Autodesk Inventor part; units mm, degrees
ref_plane "YZ Plane" through (0, 0, 0) normal (1, 0, 0) x (0, 1, 0)
ref_plane "XZ Plane" through (0, 0, 0) normal (0, 1, 0) x (-1, 0, 0)
ref_plane "XY Plane" through (0, 0, 0) normal (0, 0, 1) x (1, 0, 0)
sketch "Sketch1" plane through (0, 0, 0) normal (0, 1, 0) x (-1, 0, 0)
  arc A0 (4.5962, 6.7175) -> (6.7175, 4.5962) centre (5.6569, 5.6569) ccw
  line L0 (5.6569, 7.7782) -> (4.5962, 6.7175)
  arc A1 (7.7782, 5.6569) -> (5.6569, 7.7782) centre (6.7175, 6.7175) ccw
  line L1 (6.7175, 4.5962) -> (7.7782, 5.6569)
  circle A2 centre (0, 0) radius 3
  circle A3 centre (0, -124.0736) radius 1.5
  circle A4 centre (0, -145.2868) radius 4
  arc A5 (-4.5962, -6.7175) -> (-6.7175, -4.5962) centre (-5.6569, -5.6569) ccw
  line L2 (-5.6569, -7.7782) -> (-4.5962, -6.7175)
  arc A6 (-7.7782, -5.6569) -> (-5.6569, -7.7782) centre (-6.7175, -6.7175) ccw
  line L3 (-6.7175, -4.5962) -> (-7.7782, -5.6569)
  line L4 (-20, 5.4953) -> (-20, -6.6667)
  arc A7 (-20, -6.6667) -> (-18, -12.6667) centre (-10, -6.6667) ccw
  line L5 (-18, -12.6667) -> (-14.5, -17.3333)
  arc A8 (-12.5, -23.3333) -> (-14.5, -17.3333) centre (-22.5, -23.3333) ccw
  line L6 (-12.5, -23.3333) -> (-12.5, -134.321)
  arc A9 (-12.5, -134.321) -> (-12.2297, -138.6622) centre (22.5, -134.321) ccw
  line L7 (-12.2297, -138.6622) -> (-10, -156.5)
  line L8 (-10, -156.5) -> (-10, -166.5)
  line L9 (-10, -166.5) -> (0, -166.5)
  line L10 (0, -166.5) -> (0, -156.5)
  line L11 (0, -156.5) -> (10, -156.5)
  line L12 (10, -156.5) -> (12.2297, -138.6622)
  arc A10 (12.2297, -138.6622) -> (12.5, -134.321) centre (-22.5, -134.321) ccw
  line L13 (12.5, -134.321) -> (12.5, -23.3333)
  arc A11 (14.5, -17.3333) -> (12.5, -23.3333) centre (22.5, -23.3333) ccw
  line L14 (14.5, -17.3333) -> (18, -12.6667)
  arc A12 (18, -12.6667) -> (20, -6.6667) centre (10, -6.6667) ccw
  line L15 (20, -6.6667) -> (20, 5.4953)
  arc A13 (20, 5.4953) -> (16.6262, 12.9849) centre (10, 5.4953) ccw
  line L16 (16.6262, 12.9849) -> (6.6262, 21.8321)
  arc A14 (6.6262, 21.8321) -> (-6.6262, 21.8321) centre (0, 14.3426) ccw
  line L17 (-6.6262, 21.8321) -> (-16.6262, 12.9849)
  arc A15 (-16.6262, 12.9849) -> (-20, 5.4953) centre (-10, 5.4953) ccw
  arc A16 (-6.7175, 4.5962) -> (-4.5962, 6.7175) centre (-5.6569, 5.6569) ccw
  line L18 (-7.7782, 5.6569) -> (-6.7175, 4.5962)
  arc A17 (-5.6569, 7.7782) -> (-7.7782, 5.6569) centre (-6.7175, 6.7175) ccw
  line L19 (-4.5962, 6.7175) -> (-5.6569, 7.7782)
  arc A18 (6.7175, -4.5962) -> (4.5962, -6.7175) centre (5.6569, -5.6569) ccw
  line L20 (7.7782, -5.6569) -> (6.7175, -4.5962)
  arc A19 (5.6569, -7.7782) -> (7.7782, -5.6569) centre (6.7175, -6.7175) ccw
  line L21 (4.5962, -6.7175) -> (5.6569, -7.7782)
  circle A20 centre (6, -136.5) radius 1.5
  circle A21 centre (-6, -136.5) radius 1.5
  point P0 (18, -12.6667)
  point P1 (16.6262, 12.9849)
  point P2 (6.6262, 21.8321)
  point P3 (-6.6262, 21.8321)
  point P4 (-16.6262, 12.9849)
  point P5 (-18, -12.6667)
  point P6 (-14.5, -17.3333)
  point P7 (-12.5, -23.3333)
  point P8 (-12.5, -134.321)
  point P9 (-12.2297, -138.6622)
  point P10 (12.2297, -138.6622)
  point P11 (12.5, -134.321)
  point P12 (12.5, -23.3333)
  point P13 (14.5, -17.3333)
  point P14 (-6.7175, -4.5962)
  point P15 (-4.5962, -6.7175)
  point P16 (-5.6569, -7.7782)
  point P17 (-7.7782, -5.6569)
  point P18 (7.7782, 5.6569)
  point P19 (6.7175, 4.5962)
  point P20 (4.5962, 6.7175)
  point P21 (5.6569, 7.7782)
  point P22 (-5.6569, 7.7782)
  point P23 (-4.5962, 6.7175)
  point P24 (-6.7175, 4.5962)
  point P25 (-7.7782, 5.6569)
  point P26 (6.7175, -4.5962)
  point P27 (7.7782, -5.6569)
  point P28 (5.6569, -7.7782)
  point P29 (4.5962, -6.7175)
extrude "Extrusion1" add sketch "Sketch1" along normal blind 6
sketch "Sketch2" plane through (0, 6, 0) normal (0, 1, 0) x (1, 0, 0)
  line L0 (20, -5.4953) -> (20, 6.6667)
  arc A0 (20, 6.6667) -> (18, 12.6667) centre (10, 6.6667) ccw
  line L1 (18, 12.6667) -> (14.5, 17.3333)
  arc A1 (12.5, 23.3333) -> (14.5, 17.3333) centre (22.5, 23.3333) ccw
  line L2 (12.5, 23.3333) -> (12.5, 134.321)
  arc A2 (12.5, 134.321) -> (12.2297, 138.6622) centre (-22.5, 134.321) ccw
  line L3 (12.2297, 138.6622) -> (10, 156.5)
  line L4 (10, 156.5) -> (10, 166.5)
  line L5 (10, 166.5) -> (0, 166.5)
  line L6 (0, 166.5) -> (0, 156.5)
  line L7 (0, 156.5) -> (-10, 156.5)
  line L8 (-10, 156.5) -> (-12.2297, 138.6622)
  arc A3 (-12.2297, 138.6622) -> (-12.5, 134.321) centre (22.5, 134.321) ccw
  line L9 (-12.5, 134.321) -> (-12.5, 23.3333)
  arc A4 (-14.5, 17.3333) -> (-12.5, 23.3333) centre (-22.5, 23.3333) ccw
  line L10 (-14.5, 17.3333) -> (-18, 12.6667)
  arc A5 (-18, 12.6667) -> (-20, 6.6667) centre (-10, 6.6667) ccw
  line L11 (-20, 6.6667) -> (-20, -5.4953)
  arc A6 (-20, -5.4953) -> (-16.6262, -12.9849) centre (-10, -5.4953) ccw
  line L12 (-16.6262, -12.9849) -> (-6.6262, -21.8321)
  arc A7 (-6.6262, -21.8321) -> (6.6262, -21.8321) centre (0, -14.3426) ccw
  line L13 (6.6262, -21.8321) -> (16.6262, -12.9849)
  arc A8 (16.6262, -12.9849) -> (20, -5.4953) centre (10, -5.4953) ccw
  circle A9 centre (0, 0) radius 3
  circle A10 centre (0, 145.2868) radius 4
  circle A11 centre (-6, 136.5) radius 1.5
  circle A12 centre (6, 136.5) radius 1.5
  circle A13 centre (0, 124.0736) radius 1.5
  line L14 (7.7782, 5.6569) -> (6.7175, 4.5962)
  arc A14 (4.5962, 6.7175) -> (6.7175, 4.5962) centre (5.6569, 5.6569) ccw
  line L15 (4.5962, 6.7175) -> (5.6569, 7.7782)
  arc A15 (7.7782, 5.6569) -> (5.6569, 7.7782) centre (6.7175, 6.7175) ccw
  line L16 (-7.7782, -5.6569) -> (-6.7175, -4.5962)
  arc A16 (-4.5962, -6.7175) -> (-6.7175, -4.5962) centre (-5.6569, -5.6569) ccw
  line L17 (-4.5962, -6.7175) -> (-5.6569, -7.7782)
  arc A17 (-7.7782, -5.6569) -> (-5.6569, -7.7782) centre (-6.7175, -6.7175) ccw
  arc A18 (5.6569, -7.7782) -> (7.7782, -5.6569) centre (6.7175, -6.7175) ccw
  line L18 (5.6569, -7.7782) -> (4.5962, -6.7175)
  arc A19 (6.7175, -4.5962) -> (4.5962, -6.7175) centre (5.6569, -5.6569) ccw
  line L19 (6.7175, -4.5962) -> (7.7782, -5.6569)
  line L20 (-6.7175, 4.5962) -> (-7.7782, 5.6569)
  arc A20 (-5.6569, 7.7782) -> (-7.7782, 5.6569) centre (-6.7175, 6.7175) ccw
  line L21 (-5.6569, 7.7782) -> (-4.5962, 6.7175)
  arc A21 (-6.7175, 4.5962) -> (-4.5962, 6.7175) centre (-5.6569, 5.6569) ccw
  line L22 (18.6141, -15.2318) -> (8.6141, -24.079)
  arc A22 (-8.6141, -24.079) -> (8.6141, -24.079) centre (0, -14.3426) ccw
  line L23 (-8.6141, -24.079) -> (-18.6141, -15.2318)
  arc A23 (-23, -5.4953) -> (-18.6141, -15.2318) centre (-10, -5.4953) ccw
  line L24 (-23, -5.4953) -> (-23, 6.6667)
  arc A24 (-20.4, 14.4667) -> (-23, 6.6667) centre (-10, 6.6667) ccw
  line L25 (-20.4, 14.4667) -> (-12.5, 25)
  line L26 (-15.5, 23.3333) -> (-15.5, 134.321)
  arc A25 (-15.2066, 139.0343) -> (-15.5, 134.321) centre (22.5, 134.321) ccw
  line L27 (-15.2066, 139.0343) -> (-12.6483, 159.5)
  line L28 (-12.6483, 159.5) -> (-3, 159.5)
  line L29 (-3, 159.5) -> (-3, 169.5)
  line L30 (-3, 169.5) -> (13, 169.5)
  line L31 (13, 169.5) -> (13, 156.6868)
  line L32 (13, 156.6868) -> (15.2066, 139.0343)
  arc A26 (15.5, 134.321) -> (15.2066, 139.0343) centre (-22.5, 134.321) ccw
  line L33 (15.5, 134.321) -> (15.5, 23.3333)
  line L34 (12.5, 25) -> (20.4, 14.4667)
  arc A27 (23, 6.6667) -> (20.4, 14.4667) centre (10, 6.6667) ccw
  line L35 (23, 6.6667) -> (23, -5.4953)
  arc A28 (18.6141, -15.2318) -> (23, -5.4953) centre (10, -5.4953) ccw
  dimension "d2" = 3
extrude "Extrusion2" add sketch "Sketch2" against normal blind 6 contours L0 A0 L1 A1 L2 L34 A27 L35 A28 L22 A22 L23 A23 L24 A24 L25 L9 A4 L10 A5 L11 A6 L12 A7 L13 A8
sketch "Sketch3" plane through (0, 6, 0) normal (0, 1, 0) x (1, 0, 0)
  line L0 (12.5, 25) -> (12.5, 134.321)
  arc A0 (12.5, 134.321) -> (12.2297, 138.6622) centre (-22.5, 134.321) ccw
  line L1 (12.2297, 138.6622) -> (10, 156.5)
  line L2 (10, 156.5) -> (10, 166.5)
  line L3 (10, 166.5) -> (0, 166.5)
  line L4 (0, 166.5) -> (0, 156.5)
  line L5 (0, 156.5) -> (-10, 156.5)
  line L6 (-10, 156.5) -> (-12.2297, 138.6622)
  arc A1 (-12.2297, 138.6622) -> (-12.5, 134.321) centre (22.5, 134.321) ccw
  line L7 (-12.5, 134.321) -> (-12.5, 25)
  circle A2 centre (0, 0) radius 3
  circle A3 centre (0, 145.2868) radius 4
  circle A4 centre (-6, 136.5) radius 1.5
  circle A5 centre (6, 136.5) radius 1.5
  circle A6 centre (0, 124.0736) radius 1.5
  line L8 (7.7782, 5.6569) -> (6.7175, 4.5962)
  arc A7 (4.5962, 6.7175) -> (6.7175, 4.5962) centre (5.6569, 5.6569) ccw
  line L9 (4.5962, 6.7175) -> (5.6569, 7.7782)
  arc A8 (7.7782, 5.6569) -> (5.6569, 7.7782) centre (6.7175, 6.7175) ccw
  line L10 (-7.7782, -5.6569) -> (-6.7175, -4.5962)
  arc A9 (-4.5962, -6.7175) -> (-6.7175, -4.5962) centre (-5.6569, -5.6569) ccw
  line L11 (-4.5962, -6.7175) -> (-5.6569, -7.7782)
  arc A10 (-7.7782, -5.6569) -> (-5.6569, -7.7782) centre (-6.7175, -6.7175) ccw
  arc A11 (5.6569, -7.7782) -> (7.7782, -5.6569) centre (6.7175, -6.7175) ccw
  line L12 (5.6569, -7.7782) -> (4.5962, -6.7175)
  arc A12 (6.7175, -4.5962) -> (4.5962, -6.7175) centre (5.6569, -5.6569) ccw
  line L13 (6.7175, -4.5962) -> (7.7782, -5.6569)
  line L14 (-6.7175, 4.5962) -> (-7.7782, 5.6569)
  arc A13 (-5.6569, 7.7782) -> (-7.7782, 5.6569) centre (-6.7175, 6.7175) ccw
  line L15 (-5.6569, 7.7782) -> (-4.5962, 6.7175)
  arc A14 (-6.7175, 4.5962) -> (-4.5962, 6.7175) centre (-5.6569, 5.6569) ccw
  line L16 (-12.5, 25) -> (-20.4, 14.4667)
  arc A15 (-20.4, 14.4667) -> (-23, 6.6667) centre (-10, 6.6667) ccw
  line L17 (-23, 6.6667) -> (-23, -5.4953)
  arc A16 (-23, -5.4953) -> (-18.6141, -15.2318) centre (-10, -5.4953) ccw
  line L18 (-18.6141, -15.2318) -> (-8.6141, -24.079)
  arc A17 (-8.6141, -24.079) -> (8.6141, -24.079) centre (0, -14.3426) ccw
  line L19 (8.6141, -24.079) -> (18.6141, -15.2318)
  arc A18 (18.6141, -15.2318) -> (23, -5.4953) centre (10, -5.4953) ccw
  line L20 (23, -5.4953) -> (23, 6.6667)
  arc A19 (23, 6.6667) -> (20.4, 14.4667) centre (10, 6.6667) ccw
  line L21 (20.4, 14.4667) -> (12.5, 25)
  circle A20 centre (-6.7175, -6.7175) radius 3 construction
  line L22 (0, 0) -> (-8.8388, -8.8388) construction
  circle A21 centre (0, 0) radius 12.5
  dimension "d8" = 6
fillet "Fillet1" radius 10 2 edges at (12.5, 3, -25) (-12.5, 3, -25)
extrude "Extrusion3" cut sketch "Sketch3" against normal blind 6 contours A21
sketch "Sketch4" plane through (0, 6, 0) normal (0, 1, 0) x (1, 0, 0)
  circle A0 centre (0, 0) radius 12.5 construction
  circle A1 centre (0, 0) radius 12.5 construction
  line L0 (12.5, 0) -> (23, 0) construction
  line L1 (23, -5.4953) -> (23, 6.6667) construction
  circle A2 centre (0, 0) radius 17.75 construction
  line L2 (0, -12.5) -> (0, -17.75) construction
  line L3 (-12.5, 0) -> (-17.75, 0) construction
  line L4 (0, 12.5) -> (0, 17.75) construction
  circle A3 centre (17.75, 0) radius 1.5
  circle A4 centre (0, 17.75) radius 1.5
  circle A5 centre (-17.75, 0) radius 1.5
  circle A6 centre (0, -17.75) radius 1.5
  dimension "d11" = 3
  dimension "d14" = 360
extrude "Extrusion4" cut sketch "Sketch4" against normal up to next
sketch "Sketch5" plane through (0, 6, 0) normal (0, 1, 0) x (1, 0, 0)
  point P0 (0, 0)
properties part number "mod arms"
Can you work these out from the model? Positions are in its coordinate system, mm. A direction names the side the tool comes from. Round coordinates to 2 decimals unless told otherwise and drop trailing zeros. Write each loop counter-clockwise with the first axis right and the second up, starting at its lowest first coordinate (ties: lowest second). Pieces come first, ordered by that corner, then holes. Notation, with made-up numbers: (-14, 51) -> (11, 51) arc R20 ccw to (11, 66) -> close; hole circle Ø5 at (70, 49.25). An arc over 180 degrees is marked (long way). One line per question, with ' | ' between items. Start each with the question number.
1) On a 3-axis mill with a long thin cutter (end or side, diameter ignored), from which of +Z, -Z, +X, -X, +Y, -Y can I reach the whole of each face in a straight line? I mean faces 1 (the flat face through (-5, 3, -156.5)), 2 (the flat face through (12.5, 3, -81)), 3 (the flat face through (-13.54, 3.04, 19.72)). Say none if no direction works.
2) I need wall thicknesses on line 1 (X direction, y = 1.6, z = 0); line 2 (Z direction, x = -6, y = 2.35); line 3 (X direction, y = 4.35, z = -136.5). Which ranges of each line are inside material? Lowest first, please. Write a range as [from, to].
3) I'm going to push flat-ended pins straight in: P1, Ø1.5, axis at x = 15, y = 1.5, coming from the +Z side; P2, Ø3, axis at y = 2.5, z = -163.5, coming from the -X side; P3, Ø2.5, axis at x = 6, z = -136.5, coming from the +Y side; P4, Ø3, axis at x = -4, y = 4, coming from the -Z side. Where does each tip first touch, or does it pass through?
4) If we mould it in two halves opening along X, with no side actions, what happens to faces 4 (the cylindrical face through (-6, 3, -138)), 5 (the flat face through (0, 3, -162)), 6 (the cylindrical face through (0.521, 2.958, -149.253)), 7 (the flat face through (10, 3, -161))? For each: released by +X, released by -X, zero draft, split by the parting line, or undercut.
5) Suppose I cut it at A-A on y = 3.9. Count the separate pieces of the cut face and the enclosed holes in it, then the cut area to 3 significant figures.
6) Suppose I cut it at B-B on z = -112. Write out the boundary of the cut face in (x, y).
Return value:
1) face 1: -Z, -X, +Y, -Y | face 2: -Z, +X, +Y, -Y | face 3: +Z, -X, +Y, -Y
2) line 1: x = [-23, -19.25], [-16.25, -12.5], [12.5, 16.25], [19.25, 23] | line 2: z = [-156.5, -138], [-135, -10.97], [10.97, 25.88] | line 3: x = [-12.43, -7.5], [-4.5, 4.5], [7.5, 12.43]
3) P1: stops at z = 19.09 | P2: stops at x = 0 | P3: passes through | P4: stops at z = -156.5
4) face 4: undercut | face 5: released by -X | face 6: undercut | face 7: released by +X
5) separate pieces: 1 | enclosed holes: 9 | area: 4,700 mm2
6) outline: (-12.5, 0) -> (12.5, 0) -> (12.5, 6) -> (-12.5, 6) -> close
